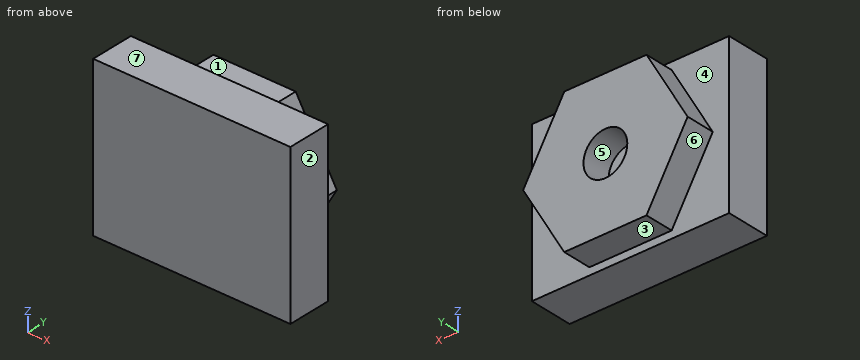
from build123d import *

# Parameters (mm, degrees)
SKETCH_1_W          = 54
SKETCH_1_H          = 43
EXTRUDE_1_DEPTH     = 12
SKETCH_2_R          = 1.55
EXTRUDE_2_DEPTH     = 8
SKETCH_4_R          = 6
CUT_EXTRUDE_2_DEPTH = 8


with BuildPart() as part:
    # 草图1 → 凸台-拉伸1 (new body)
    with BuildSketch(Plane(origin=(0, 0, 0), x_dir=(1, 0, 0), z_dir=(0, 1, 0))):
        Rectangle(SKETCH_1_W, SKETCH_1_H)
    extrude(amount=EXTRUDE_1_DEPTH)

    # 草图2 → 凸台-拉伸2 (add)
    with BuildSketch(Plane(origin=(0, 12, 0), x_dir=(1, 0, 0), z_dir=(0, 1, 0))):
        Polygon((-22.516660498, 0), (-11.258330249, -19.5), (11.258330249, -19.5), (22.516660498, 0), (11.258330249, 19.5), (-11.258330249, 19.5), align=None)
        with Locations(Location((0, 0, 0), (0, 0, 270))):
            Circle(SKETCH_2_R, mode=Mode.SUBTRACT)
    extrude(amount=EXTRUDE_2_DEPTH)

    # 草图4 → 切除-拉伸2 (cut)
    with BuildSketch(Plane(origin=(0, 20, 0), x_dir=(1, 0, 0), z_dir=(0, 1, 0))):
        with Locations(Location((0, 0, 0), (0, 0, 270))):
            Circle(SKETCH_4_R)
    extrude(amount=-CUT_EXTRUDE_2_DEPTH, mode=Mode.SUBTRACT)


solid = part.part
Work out the finished part from the listing and answer in its coordinate system (mm). Face numbers are marked on the shaded views. A direction names the side the tool comes from. Round coordinates to 2 decimals unless told otherwise and drop trailing zeros. Order: outer loops, then holes, each group sorted by start corner. A loop starts at its lowest first (then second) coordinate and runs counter-clockwise, first axis right, second up. Notation, with made-up numbers: M -20,11.25 L 0,11.25 A5 cw 0,15.25 Z; hole C -27,84.25 d8. An arc over 180 degrees is marked long. Put each result on its own line as item: value. Start each with the question number.
Q1. For a pull along Z with two mould halves and no side action, classify the marked faces 5, 6 and 7 as pulls with the +Z half, pulls with the -Z half, needs draft (parallel to the pull), parting line crosses it, or undercut.
Q2. Section A-A, the plane y = 18 is taken. Write down the section's boundary in (x, z), and give its area (3 significant figures).
Q3. Flat-ended cylindrical pins translate along their axes: pin 1 (8 mm diameter, centred on y = 15.5, z = -10, fed in from -X); pin 2 (3.5 mm diameter, centred on x = 1.5, z = 1.5, fed in from +Y); pin 3 (4 mm diameter, centred on x = -3, y = 16.5, fed in from -Z). Find the tip coordinate at first contact, or state that the pin passes through.
Q4. Straight lines are drawn through the part: L1, parallel to X at y = 17.5, z = 0; L2, parallel to Y at x = -21.5, z = 7; L3, parallel to X at y = 16.5, z = -3. For each, find the intervals that lie inside material, in ascending order. Write a range as [from, to].
Q5. A tool of negligible diameter and unlimited length cuts with its end or side. For the marked faces 1, 2, 3 and 4, from which of +Z, -Z, +X, -X, +Y, -Y can it reach the whole face along a straight path? Write none if from no direction.
Q6. Section C-C, the plane z = 13.5 is taken. Write down the section's boundary in (x, y).
Q7. Section D-D, the plane x = -18.5 is taken. Write down the section's boundary in (y, z).
Q8. Section B-B, the plane x = 0 is taken. Write down the section's boundary in (y, z).
Findings below:
1. face 5: undercut
1. face 6: pulls with the -Z half
1. face 7: pulls with the +Z half
2. outline: M -22.52,0 L -11.26,-19.5 L 11.26,-19.5 L 22.52,0 L 11.26,19.5 L -11.26,19.5 Z; hole C 0,0 d12
2. area: 1,200 mm^2
3. pin 1: stops at x = -27
3. pin 2: stops at y = 12
3. pin 3: stops at z = -19.5
4. L1: x = [-22.52, -6], [6, 22.52]
4. L2: y = [0, 12]
4. L3: x = [-20.78, -5.2], [5.2, 20.78]
5. face 1: +Z, +X, -X, +Y
5. face 2: +Z, -Z, +X, +Y, -Y
5. face 3: -Z, +X, -X, +Y
5. face 4: +Y
6. outline: M -27,0 L 27,0 L 27,12 L 14.72,12 L 14.72,20 L -14.72,20 L -14.72,12 L -27,12 Z
7. outline: M 0,-21.5 L 12,-21.5 L 12,-6.96 L 20,-6.96 L 20,6.96 L 12,6.96 L 12,21.5 L 0,21.5 Z
8. outline: M 0,-21.5 L 12,-21.5 L 12,-19.5 L 20,-19.5 L 20,-6 L 12,-6 L 12,6 L 20,6 L 20,19.5 L 12,19.5 L 12,21.5 L 0,21.5 Z
